Check sheet for the drawn part. Datum: minimum x, y, z corner. Units: mm. Round coordinates to 2 decimals unless told otherwise and drop trailing zeros. Order: outer loops, then holes, each group sorted by start corner. A loop starts at its lowest first (then second) coordinate and runs counter-clockwise, first axis right, second up. Notation, with made-up numbers: (-10, 75.25) -> (47, 75.25) arc R26 cw to (47, 105.25) -> close; hole circle Ø2 at (1, 2.5). An arc over 180 degrees is marked (long way). Answer in a Markdown table with one row per item.
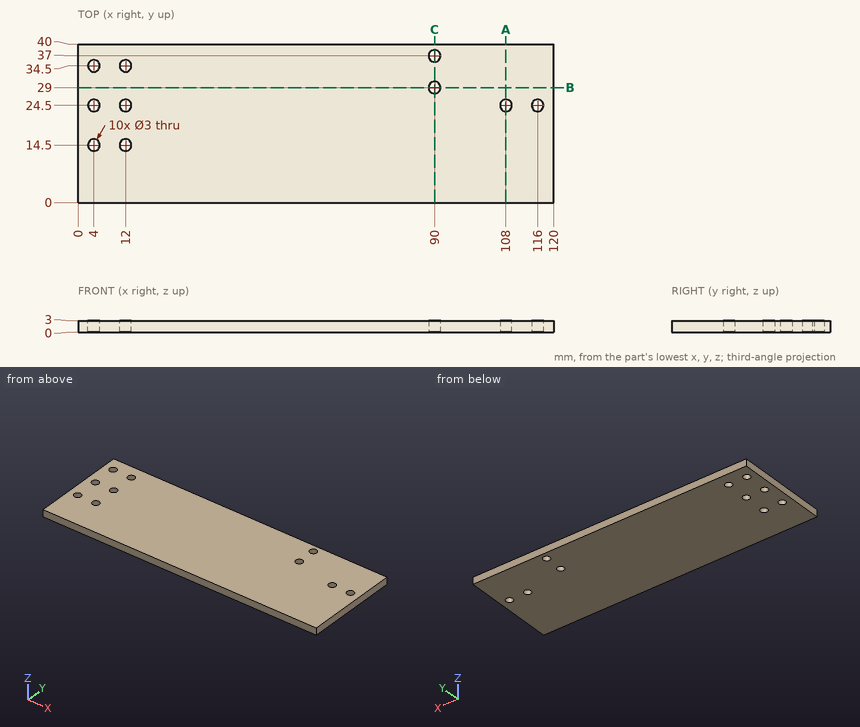
(1) Depth check by flat-ended pin: pin 1 Ø1.8 at (x, y) = (90, 37) entering from +Z. Enter the tip coordinate at first touch or a pass-through.
Solutions:
| item | result |
|---|---|
| pin 1 | through |
(2) Section check A-A on x = 108. Record the boundary of the cut face in (y, z).
Solutions:
| item | result |
|---|---|
| outline | (0, 0) -> (23, 0) -> (23, 3) -> (0, 3) -> close; (26, 0) -> (40, 0) -> (40, 3) -> (26, 3) -> close |
(3) Scan lines: probe 1 along X at (y, z) = (14.5, 1.55); probe 2 along X at (y, z) = (23.5, 2.6); probe 3 along X at (y, z) = (30, 0.2). Record each from-to range of solid material in increasing order. Write a range as from..to.
Solutions:
| item | result |
|---|---|
| probe 1 | 0..2.5, 5.5..10.5, 13.5..120 |
| probe 2 | 0..2.88, 5.12..10.88, 13.12..106.88, 109.12..114.88, 117.12..120 |
| probe 3 | 0..88.88, 91.12..120 |
(4) Section check B-B on y = 29. Record the boundary of the cut face in (x, z), plus the area to 3 significant figures.
Solutions:
| item | result |
|---|---|
| outline | (0, 0) -> (88.5, 0) -> (88.5, 3) -> (0, 3) -> close; (91.5, 0) -> (120, 0) -> (120, 3) -> (91.5, 3) -> close |
| area | 351 mm^2 |
(5) Section check C-C on x = 90. Record the boundary of the cut face in (y, z), plus the area to 3 significant figures.
Solutions:
| item | result |
|---|---|
| outline | (0, 0) -> (27.5, 0) -> (27.5, 3) -> (0, 3) -> close; (30.5, 0) -> (35.5, 0) -> (35.5, 3) -> (30.5, 3) -> close; (38.5, 0) -> (40, 0) -> (40, 3) -> (38.5, 3) -> close |
| area | 102 mm^2 |
